from build123d import *

# Parameters (mm, degrees)
F0_W     = 76.2
F0_H     = 508
F1_DEPTH = 50.8
F3_DEPTH = 50.801
F5_DEPTH = 50.801
F7_DEPTH = 50.801


with BuildPart() as f1:
    # F0 (on Front) → F1 (new body)
    with BuildSketch(Plane.XZ):
        Rectangle(F0_W, F0_H)
    extrude(amount=F1_DEPTH)

    # F2 (on face) → F3 (cut, through all)
    with BuildSketch(Plane.XZ.offset(50.8)):
        Polygon((38.1, -254), (-38.1, -223.2132015914), (-38.1, -254), align=None)
        Polygon((38.1, 223.2132015914), (38.1, 254), (-38.1, 254), align=None)
    extrude(amount=-F3_DEPTH, mode=Mode.SUBTRACT)

    # F4 (on face) → F5 (cut, through all)
    with BuildSketch(Plane.XZ.offset(50.8)):
        Polygon((-26.324765047, 201.3016269516), (-38.1, 254), (-38.1, 206.059130688), align=None)
        Polygon((38.1, 175.2723322793), (38.1, 223.2132015914), (26.324765047, 180.0298360157), align=None)
    extrude(amount=-F5_DEPTH, mode=Mode.SUBTRACT)

    # F6 (on face) → F7 (cut, through all)
    with BuildSketch(Plane.XZ.offset(50.8)):
        Polygon((-14.549530094, -232.7282090641), (-38.1, 129.859130688), (-38.1, -223.2132015914), align=None)
    extrude(amount=-F7_DEPTH, mode=Mode.SUBTRACT)


solid = f1.part
The model under review builds one solid part; all positions refer to its coordinate system, in mm. A direction names the side the tool comes from. Give positions to 0.01 mm unless a question says otherwise; leave off trailing zeros. Write each loop counter-clockwise with the first axis right and the second up, starting at its lowest first coordinate (ties: lowest second). Pieces come first, ordered by that corner, then holes.
1. Wall thickness on L1, parallel to X at y = -18.5, z = -111.5; L2, parallel to Z at x = 10, y = -2.5; L3, parallel to Z at x = -3.5, y = -25: over which ranges is each line inside the solid? List them lowest first.
2. Add section A-A, the plane y = -22.5. Write out the cut boundary in (x, z).
3. For P1, Ø3, axis at x = -6.5, y = -45.5, coming from the +Z side; P2, Ø3, axis at x = -16, y = -42.5, coming from the +Z side; P3, Ø2, axis at x = 23, y = -34, coming from the +Z side; P4, Ø1, axis at x = -20.5, z = -150, coming from the -Y side, all flat-tipped, find the tip position at first contact; note any pin that passes through.
4. Add section B-B, the plane z = 219. Write out the cut boundary in (x, y), plus the area to 3 significant figures.
5. Add section C-C, the plane x = 12. Write out the cut boundary in (y, z).
6. Tool access review of faces 5 (the flat face through (-1, 0, 4)), 6 (the flat face through (32.13, -25.756, 177.684)): name each direction out of +Z, -Z, +X, -X, +Y, -Y from which nothing blocks a thin tool from reaching the whole face with its end or side.
7. Draft analysis for pull direction Z (two halves, no side actions). For faces 1 (the flat face through (-0.53, -25.76, 238.82)), 2 (the flat face through (-32.13, -25.76, 227.28)), 3 (the flat face through (12.14, -25.76, -243.51)), 4 (the flat face through (-32.29, -25.76, 203.71)), state which applies: +Z half, -Z half, draft (parallel to the pull), parting line (faces both ways), or undercut.
Worked answers:
1. L1: x = -22.42 to 38.1
1. L2: z = -242.65 to 234.57
1. L3: z = -237.19 to 240.02
2. outline: (-38.1, 129.86) - (-14.55, -232.73) - (38.1, -254) - (38.1, 175.27) - (26.32, 180.03) - (38.1, 223.21) - (-38.1, 254) - (-26.32, 201.3) - (-38.1, 206.06) - close
3. P1: stops at z = 241.84
3. P2: stops at z = 245.68
3. P3: stops at z = 229.72
3. P4: passes through
4. outline: (-30.28, -50.8) - (36.95, -50.8) - (36.95, 0) - (-30.28, 0) - close
4. area: 3,420 mm2
5. outline: (-50.8, -243.45) - (0, -243.45) - (0, 233.76) - (-50.8, 233.76) - close
6. face 5: +Z, -Z, +X, -X, +Y
6. face 6: +X, +Y, -Y
7. face 1: +Z half
7. face 2: undercut
7. face 3: -Z half
7. face 4: undercut
